from build123d import *

# Parameters (mm, degrees)
SKETCH1_R            = 18
SKETCH1_R_2          = 5
BODY_DEPTH           = 5
OBJECTIVE_RING_SIZE  = 6
OBJECTIVE_RING_SIZE2 = 4.5
SKETCH6_R            = 1.6
BOLTS_DEPTH          = 10
BOLTS_DEPTH_BACK     = 10
SKETCH8_R            = 3
SKETCH8_R_2          = 1.6
WASH_DEPTH           = 0.5
SKETCH9_W            = 8
SKETCH9_H            = 12
SPE_DEPTH            = 10
SPE_DEPTH_BACK       = 9.5
SPE_FILLET_R         = 1


with BuildPart() as part:
    # Sketch1 → Body (new body)
    with BuildSketch(Plane(origin=(0, 0, 0), x_dir=(1, 0, 0), z_dir=(0, 1, 0))):
        Circle(SKETCH1_R)
        Circle(SKETCH1_R_2, mode=Mode.SUBTRACT)
    extrude(amount=BODY_DEPTH)

    # Objective_ring
    objective_ring_edges = [part.edges().sort_by_distance(p)[0] for p in [
        (-5, 5, 0),
    ]]
    objective_ring_side = [part.faces().sort_by_distance(p)[0] for p in [
        (-17.490883118, 5, 0),
    ]]
    chamfer(objective_ring_edges, length=OBJECTIVE_RING_SIZE, length2=OBJECTIVE_RING_SIZE2, reference=objective_ring_side[0])

    # Sketch6 → Bolts (cut, two sides)
    with BuildSketch(Plane(origin=(0, 5, 0), x_dir=(1, 0, 0), z_dir=(0, 1, 0))) as bolts_sk:
        with Locations((-10.253048327, 10.253048327)):
            Circle(SKETCH6_R)
        with Locations((-10.253048327, -10.253048327)):
            Circle(SKETCH6_R)
        with Locations((10.253048327, -10.253048327)):
            Circle(SKETCH6_R)
        with Locations((10.253048327, 10.253048327)):
            Circle(SKETCH6_R)
    extrude(amount=BOLTS_DEPTH, mode=Mode.SUBTRACT)
    extrude(bolts_sk.sketch, amount=-BOLTS_DEPTH_BACK, mode=Mode.SUBTRACT)

    # Sketch8 → Wash (add)
    with BuildSketch(Plane(origin=(0, 5, 0), x_dir=(1, 0, 0), z_dir=(0, 1, 0))):
        with Locations((-10.253048327, 10.253048327)):
            Circle(SKETCH8_R)
        with Locations((-10.253048327, 10.253048327)):
            Circle(SKETCH8_R_2, mode=Mode.SUBTRACT)
        with Locations((10.253048327, 10.253048327)):
            Circle(SKETCH8_R)
        with Locations((10.253048327, 10.253048327)):
            Circle(SKETCH8_R_2, mode=Mode.SUBTRACT)
        with Locations((10.253048327, -10.253048327)):
            Circle(SKETCH8_R)
        with Locations((10.253048327, -10.253048327)):
            Circle(SKETCH8_R_2, mode=Mode.SUBTRACT)
        with Locations((-10.253048327, -10.253048327)):
            Circle(SKETCH8_R)
        with Locations((-10.253048327, -10.253048327)):
            Circle(SKETCH8_R_2, mode=Mode.SUBTRACT)
    extrude(amount=WASH_DEPTH)

    # Sketch9 → SPE (cut, two sides)
    with BuildSketch(Plane(origin=(0, 5, 0), x_dir=(1, 0, 0), z_dir=(0, 1, 0))) as spe_sk:
        with Locations((-18, 0)):
            Rectangle(SKETCH9_W, SKETCH9_H)
    extrude(amount=SPE_DEPTH, mode=Mode.SUBTRACT)
    extrude(spe_sk.sketch, amount=-SPE_DEPTH_BACK, mode=Mode.SUBTRACT)

    # SPE_Fillet
    spe_fillet_edges = [part.edges().sort_by_distance(p)[0] for p in [
        (-16.970562748, 2.5, 6),
        (-16.970562748, 2.5, -6),
    ]]
    fillet(spe_fillet_edges, radius=SPE_FILLET_R)


solid = part.part
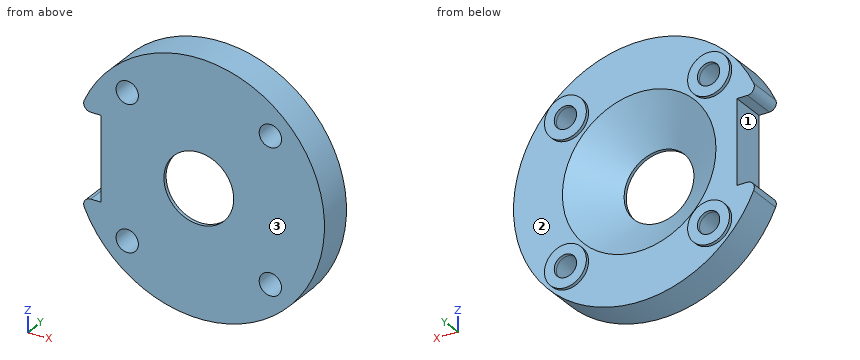
Verification items for the finished model (mm, model axes). Face numbers are marked on the shaded views. A direction names the side the tool comes from. Coordinates: 2 decimals unless noted, no trailing zeros. Order: outer loops, then holes, each group sorted by start corner. A loop starts at its lowest first (then second) coordinate and runs counter-clockwise, first axis right, second up.
1. Scan lines: line 1 (Z direction, x = 9, y = 1.8); line 2 (X direction, y = 1.2, z = 10.5); line 3 (Y direction, x = 8.5, z = -14). Record each from-to range of solid material in increasing order.
Results found:
line 1: z = -15.59 to -11.25, -9.26 to 9.26, 11.25 to 15.59
line 2: x = -14.62 to -11.83, -8.67 to 8.67, 11.83 to 14.62
line 3: y = 0 to 5
2. Go/stop test with flat-tipped pins: pin 1 Ø3.5 at (x, z) = (-10.25, -10.25) entering from +Y; pin 2 Ø1.2 at (x, y) = (-14.5, 3) entering from -Z; pin 3 Ø3 at (y, z) = (3.5, -13) entering from -X; pin 4 Ø11.5 at (x, z) = (0, 0) entering from +Y. Record where each tip stops, or that it passes through.
Results found:
pin 1: stops at y = 5.5
pin 2: stops at z = -11.44
pin 3: stops at x = -13.85
pin 4: stops at y = 1.06
3. Sectioned sample at A-A, the plane z = 0. Record the cut outline in (x, y).
Results found:
outline: (-14, 0) - (-5, 0) - (-5, 0.5) - (-11, 5) - (-14, 5) - close; (5, 0) - (18, 0) - (18, 5) - (11, 5) - (5, 0.5) - close
4. Sectioned sample at C-C, the plane y = 3.2. Record the cut outline in (x, z), and give its area (3 significant figures).
Results found:
outline: (-16.4, -7.41) arc R18 ccw (long way) to (-16.4, 7.41) arc R1 ccw to (-15.49, 6) - (-14, 6) - (-14, -6) - (-15.49, -6) arc R1 ccw to start; hole circle Ø3.2 at (-10.25, -10.25); hole circle Ø3.2 at (-10.25, 10.25); hole circle Ø17.2 at (0, 0); hole circle Ø3.2 at (10.25, -10.25); hole circle Ø3.2 at (10.25, 10.25)
area: 708 mm2
5. Set-up check for the marked faces 1, 2 and 3: record each of +Z, -Z, +X, -X, +Y, -Y from which the full face is reachable in a straight line by a thin tool's end or side.
Results found:
face 1: -X, +Y, -Y
face 2: +Y
face 3: +Z, -Z, +X, -X, -Y
6. Sectioned sample at B-B, the plane x = 0. Record the cut outline in (y, z), and give its area (3 significant figures).
Results found:
outline: (0, -18) - (5, -18) - (5, -11) - (0.5, -5) - (0, -5) - close; (0, 5) - (0.5, 5) - (5, 11) - (5, 18) - (0, 18) - close
area: 103 mm2
7. Sectioned sample at D-D, the plane x = -12.5. Record the cut outline in (y, z), and give its area (3 significant figures).
Results found:
outline: (0, -12.95) - (5, -12.95) - (5, -12.24) - (5.5, -12.24) - (5.5, -8.27) - (5, -8.27) - (5, 8.27) - (5.5, 8.27) - (5.5, 12.24) - (5, 12.24) - (5, 12.95) - (0, 12.95) - close
area: 133 mm2
